Check sheet for the modelled part. Datum: model origin and axes. Units: mm. A direction names the side the tool comes from. Round coordinates to 2 decimals unless told otherwise and drop trailing zeros. Loops run counter-clockwise (first coordinate to the right, second up) from the corner with the lowest first, then second, coordinate; pieces in that order, holes last. Notation, with made-up numbers: (38.25, 6.5) - (88.25, 6.5) arc R24 ccw to (88.25, 42.5) - close; hole circle Ø9 at (19.25, -32.5). An arc over 180 degrees is marked (long way). Return JSON: item names as keys, results as strings.
from build123d import *

# Parameters (mm, degrees)
F3_DEPTH = 12.7
F1_R     = 1.5875
F4_DEPTH = 39.37
F5_DEPTH = 8.382
F6_R     = 5.08
F7_R     = 5.08
F8_R     = 5.08


with BuildPart() as f3:
    # F0 (on Front) → F3 (new body, symmetric)
    with BuildSketch(Plane.XZ):
        Polygon((0, 25.4), (0, 0), (2.54, 0), (2.54, 22.86), (25.4, 22.86), (25.4, 25.4), align=None)
    extrude(amount=F3_DEPTH, both=True)

    # F1 (on Top) → F4 (cut)
    with BuildSketch(Plane.XY):
        with Locations((19.05, 6.35)):
            Circle(F1_R)
        with Locations((19.05, -6.35)):
            Circle(F1_R)
    extrude(amount=F4_DEPTH, mode=Mode.SUBTRACT)

    # F2 (on Right) → F5 (cut)
    with BuildSketch(Plane.YZ):
        with BuildLine():
            ThreePointArc((7.9375, 6.35), (5.227468, 7.472532), (6.35, 4.7625))
            ThreePointArc((6.35, 4.7625), (7.472532, 5.227468), (7.9375, 6.35))
        make_face()
        with BuildLine():
            ThreePointArc((-4.7625, 6.35), (-7.472532, 7.472532), (-6.35, 4.7625))
            ThreePointArc((-6.35, 4.7625), (-5.227468, 5.227468), (-4.7625, 6.35))
        make_face()
    extrude(amount=F5_DEPTH, mode=Mode.SUBTRACT)

    # F6
    f6_edges = [f3.edges().sort_by_distance(p)[0] for p in [
        (25.4, -12.7, 24.13),
        (25.4, 12.7, 24.13),
        (1.27, -12.7, 0),
        (1.27, 12.7, 0),
    ]]
    fillet(f6_edges, radius=F6_R)

    # F7
    f7_edges = [f3.edges().sort_by_distance(p)[0] for p in [
        (0, 0, 25.4),
    ]]
    fillet(f7_edges, radius=F7_R)

    # F8
    f8_edges = [f3.edges().sort_by_distance(p)[0] for p in [
        (2.54, 0, 22.86),
    ]]
    fillet(f8_edges, radius=F8_R)


solid = f3.part
Q1. Sectioned sample at D-D (y = 5.5). Enter the section's corners in (x, z), plus the area to 3 significant figures.
Answer key:
{"outline": "(0, 0) - (2.54, 0) - (2.54, 5.01) - (0, 5.01) - close; (0, 7.69) - (2.54, 7.69) - (2.54, 17.78) arc R5.08 cw to (7.62, 22.86) - (17.71, 22.86) - (17.71, 25.4) - (5.08, 25.4) arc R5.08 ccw to (0, 20.32) - close; (20.39, 22.86) - (25.4, 22.86) - (25.4, 25.4) - (20.39, 25.4) - close", "area": "109 mm²"}
Q2. Depth check by flat-ended pin: P1, Ø10, axis at x = 8.5, y = -4.5, coming from the -Z side; P2, Ø5.5, axis at x = 16.5, y = -3.5, coming from the -Z side; P3, Ø12, axis at y = 6, z = 9, coming from the +X side. Enter the tip coordinate at first touch or a pass-through.
Answer key:
{"P1": "stops at z = 20.75", "P2": "stops at z = 22.86", "P3": "stops at x = 2.54"}
Q3. Sectioned sample at A-A (x = 19.05). Enter the section's corners in (y, z), plus the area to 3 significant figures.
Answer key:
{"outline": "(-12.7, 22.86) - (-7.94, 22.86) - (-7.94, 25.4) - (-12.7, 25.4) - close; (-4.76, 22.86) - (4.76, 22.86) - (4.76, 25.4) - (-4.76, 25.4) - close; (7.94, 22.86) - (12.7, 22.86) - (12.7, 25.4) - (7.94, 25.4) - close", "area": "48.4 mm²"}
Q4. Sectioned sample at C-C (z = 11.5). Enter the section's corners in (x, y).
Answer key:
{"outline": "(0, -12.7) - (2.54, -12.7) - (2.54, 12.7) - (0, 12.7) - close"}
Q5. Draft check along Y on faces 1 (the face through (3.989, -0.178, 21.332)), 2 (the face through (17.464, 6.42, 24.112)), 3 (the face through (3, 12.7, 21)). Enter one of: released by +Y, released by -Y, zero draft, split by the parting line, or undercut.
Answer key:
{"face 1": "zero draft", "face 2": "undercut", "face 3": "released by +Y"}
Q6. Sectioned sample at B-B (y = -7.25). Enter the section's corners in (x, z).
Answer key:
{"outline": "(0, 0) - (2.54, 0) - (2.54, 5.04) - (0, 5.04) - close; (0, 7.66) - (2.54, 7.66) - (2.54, 17.78) arc R5.08 cw to (7.62, 22.86) - (17.74, 22.86) - (17.74, 25.4) - (5.08, 25.4) arc R5.08 ccw to (0, 20.32) - close; (20.36, 22.86) - (25.4, 22.86) - (25.4, 25.4) - (20.36, 25.4) - close"}
Q7. Scan lines: probe 1 along Y at (x, z) = (1.7, 6.35); probe 2 along Z at (x, y) = (9.5, -11.5); probe 3 along X at (y, z) = (8.5, 7.5). Record each from-to range of solid material in increasing order. Write a range as [from, to].
Answer key:
{"probe 1": "y = [-12.7, -7.94], [-4.76, 4.76], [7.94, 12.7]", "probe 2": "z = [22.86, 25.4]", "probe 3": "x = [0, 2.54]"}
Q8. Tool access check on faces 4 (the face through (16, 0, 22.86)), 5 (the face through (17.464, -6.28, 24.112)). Record the directions out of +Z, -Z, +X, -X, +Y, -Y that give a thin tool (end or side, any length) a straight path to the whole face; none if there is none.
Answer key:
{"face 4": "-Z, +X, +Y, -Y", "face 5": "+Z, -Z"}
